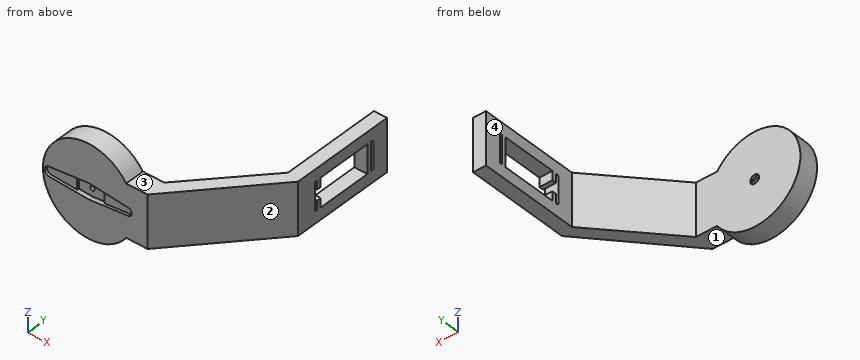
from build123d import *

# Parameters (mm, degrees)
EXTRUDE_1_DEPTH        = 15
EXTRUDE_2_DEPTH        = 40
F_1_4_BASE_D           = 3.4
F_1_4_BASE_CBORE_D     = 6.7
F_1_4_BASE_CBORE_DEPTH = 1.65
SKETCH_11_W            = 22
SKETCH_11_H            = 42
CUT_EXTRUDE_1_DEPTH    = 32
CUT_EXTRUDE_3_DEPTH    = 2
CUT_EXTRUDE_4_DEPTH    = 3.5
CUT_EXTRUDE_5_DEPTH    = 20
SKETCH_22_W            = 8
SKETCH_22_H            = 3.3
CUT_EXTRUDE_6_DEPTH    = 20


with BuildPart() as part:
    # 草图1 → 凸台-拉伸1 (new body)
    with BuildSketch(Plane(origin=(0, 0, 0), x_dir=(1, 0, 0), z_dir=(0, 1, 0))):
        with BuildLine():
            Line((45.055476805, 20), (28.722813233, 20))
            ThreePointArc((28.722813233, 20), (33.393850206, 10.480971731), (35, 0))
            ThreePointArc((35, 0), (33.393850206, -10.480971731), (28.722813233, -20))
            Line((28.722813233, -20), (45.055476805, -20))
            Line((45.055476805, -20), (45.055476805, 20))
        make_face()
        with BuildLine():
            Line((0.055476805, -20), (0.055476805, 20))
            Line((0.055476805, 20), (28.722813233, 20))
            ThreePointArc((28.722813233, 20), (-35, 0), (28.722813233, -20))
            Line((28.722813233, -20), (0.055476805, -20))
        make_face()
        with BuildLine():
            Line((28.722813233, 20), (0.055476805, 20))
            Line((0.055476805, 20), (0.055476805, -20))
            Line((0.055476805, -20), (28.722813233, -20))
            ThreePointArc((28.722813233, -20), (33.393850206, -10.480971731), (35, 0))
            ThreePointArc((35, 0), (33.393850206, 10.480971731), (28.722813233, 20))
        make_face()
    extrude(amount=EXTRUDE_1_DEPTH)

    # 草图2 → 凸台-拉伸2 (add)
    with BuildSketch(Plane.XY.offset(20)):
        Polygon((45.055476805, 0), (103.81943921, 66.228799241), (103.81943921, 146.228799241), (93.81943921, 146.228799241), (93.81943921, 69.009357532), (45.055476805, 15), align=None)
    extrude(amount=-EXTRUDE_2_DEPTH)

    # 1/4 六角头螺钉的柱形沉头孔base (through all)
    with Locations(Plane(origin=(0, 15, 0), x_dir=(1, 0, 0), z_dir=(0, 1, 0))):
        with Locations((0, 0)):
            CounterBoreHole(F_1_4_BASE_D / 2, F_1_4_BASE_CBORE_D / 2, F_1_4_BASE_CBORE_DEPTH)

    # 草图11 → 切除-拉伸1 (cut)
    with BuildSketch(Plane(origin=(103.81943921, 0, 0), x_dir=(0, 0, -1), z_dir=(1, 0, 0))):
        with Locations((0, 107.618799241)):
            Rectangle(SKETCH_11_W, SKETCH_11_H)
    extrude(amount=-CUT_EXTRUDE_1_DEPTH, mode=Mode.SUBTRACT)

    # 草图19 → 切除-拉伸3 (cut)
    with BuildSketch(Plane.XZ):
        with BuildLine():
            Line((-29.938978194, 2.983548036), (0, 6))
            Line((0, 6), (29.925496738, 2.977040035))
            ThreePointArc((29.925496738, 2.977040035), (32.999946297, -0.039985046), (29.889613095, -3.020003134))
            Line((29.889613095, -3.020003134), (0, -6))
            Line((0, -6), (-30.07371717, -4.263466486))
            ThreePointArc((-30.07371717, -4.263466486), (-33.623512821, -0.572707651), (-29.938978194, 2.983548036))
        make_face()
    extrude(amount=-CUT_EXTRUDE_3_DEPTH, mode=Mode.SUBTRACT)

    # 草图20 → 切除-拉伸4 (cut)
    with BuildSketch(Plane.XZ):
        Polygon((0, 6), (-10.447108364, 4.947418969), (-10.447108364, -5.396757185), (0, -6), (10.446834114, -4.958449786), (10.446834114, 4.944700515), align=None)
    extrude(amount=-CUT_EXTRUDE_4_DEPTH, mode=Mode.SUBTRACT)

    # 草图21 → 切除-拉伸5 (cut)
    with BuildSketch(Plane(origin=(103.81943921, 0, 0), x_dir=(0, 0, -1), z_dir=(1, 0, 0))):
        with BuildLine():
            Line((-10, 133.918799241), (10, 133.918799241))
            ThreePointArc((10, 133.918799241), (11, 132.918799241), (10, 131.918799241))
            Line((10, 131.918799241), (-10, 131.918799241))
            ThreePointArc((-10, 131.918799241), (-11, 132.918799241), (-10, 133.918799241))
        make_face()
        with BuildLine():
            Line((-10, 83.318799241), (10, 83.318799241))
            ThreePointArc((10, 83.318799241), (11, 82.318799241), (10, 81.318799241))
            Line((10, 81.318799241), (-10, 81.318799241))
            ThreePointArc((-10, 81.318799241), (-11, 82.318799241), (-10, 83.318799241))
        make_face()
    extrude(amount=-CUT_EXTRUDE_5_DEPTH, mode=Mode.SUBTRACT)

    # 草图22 → 切除-拉伸6 (cut)
    with BuildSketch(Plane(origin=(103.81943921, 0, 0), x_dir=(0, 0, -1), z_dir=(1, 0, 0))):
        with Locations((0, 84.968799241)):
            Rectangle(SKETCH_22_W, SKETCH_22_H)
    extrude(amount=-CUT_EXTRUDE_6_DEPTH, mode=Mode.SUBTRACT)


solid = part.part
Verification items for the finished model (mm, model axes). Face numbers are marked on the shaded views. A direction names the side the tool comes from. Coordinates: 2 decimals unless noted, no trailing zeros. Order: outer loops, then holes, each group sorted by start corner. A loop starts at its lowest first (then second) coordinate and runs counter-clockwise, first axis right, second up. Notation, with made-up numbers: M -2.75,-8 L 16.25,-8 A15 ccw 16.25,19 Z; hole C -24.5,6 d6. An arc over 180 degrees is marked long. One line per item, written item: value. Start each with the question number.
Item 1: Sectioned sample at A-A on y = 92. Record the cut outline in (x, z).
Item 2: Thickness scan on probe 1 along Z at (x, y) = (0, 9); probe 2 along Z at (x, y) = (0, 14.3); probe 3 along Y at (x, z) = (-10, -20.5). Record the ranges inside material, lowest first.
Item 3: Depth check by flat-ended pin: P1, Ø2, axis at x = -6.5, z = 26.5, coming from the -Y side; P2, Ø2, axis at x = -14, z = -1, coming from the -Y side; P3, Ø3.5, axis at x = 1, z = 1, coming from the +Y side; P4, Ø5.5, axis at x = 0, z = 0, coming from the -Y side. Enter the tip coordinate at first touch or a pass-through.
Item 4: Sectioned sample at B-B on x = -22.5. Record the cut outline in (y, z), then the cut area to 3 significant figures.
Item 5: Sectioned sample at D-D on x = 75.5. Record the cut outline in (y, z).
Item 6: Access from +Z, -Z, +X, -X, +Y, -Y to the whole of each face (thin tool, end or side, straight path). Record for the marked faces 1, 2, 3 and 4.
Item 7: Sectioned sample at C-C on z = 14. Record the cut outline in (x, y).
Calculated:
1. outline: M 93.82,-20 L 103.82,-20 L 103.82,-11 L 93.82,-11 Z; M 93.82,11 L 103.82,11 L 103.82,20 L 93.82,20 Z
2. probe 1: -35 to -1.7, 1.7 to 35
2. probe 2: -35 to -3.35, 3.35 to 35
2. probe 3: 0 to 15
3. P1: y = 0
3. P2: y = 2
3. P3: y = 13.35
3. P4: y = 3.5
4. outline: M 0,-26.81 L 15,-26.81 L 15,26.81 L 0,26.81 L 0,3.73 L 2,3.73 L 2,-4.7 L 0,-4.7 Z
4. area: 787 mm^2
5. outline: M 34.31,-20 L 48.72,-20 L 48.72,20 L 34.31,20 Z
6. face 1: -Z, +X, +Y, -Y
6. face 2: +Z, -Z, +X, -Y
6. face 3: +Z, +X, +Y, -Y
6. face 4: +Z, -Z, -X, +Y
7. outline: M -32.08,0 L 45.06,0 L 103.82,66.23 L 103.82,146.23 L 93.82,146.23 L 93.82,69.01 L 45.06,15 L -32.08,15 Z
